Geometry: final body of the model. Coordinates: model frame, mm. Round coordinates to 2 decimals unless told otherwise and drop trailing zeros. Loops run counter-clockwise (first coordinate to the right, second up) from the corner with the lowest first, then second, coordinate; pieces in that order, holes last. Notation, with made-up numbers: M 78,18 L 136,18 A22 ccw 136,25 Z; hole C 69,-30 d3. An arc over 180 degrees is marked long. Answer as a JSON object with one key per item and string values.
from build123d import *

# Parameters (mm, degrees)
SKETCH2_R           = 5
BOSS_EXTRUDE1_DEPTH = 10


with BuildPart() as part:
    # Sketch2 → Boss-Extrude1 (new body)
    with BuildSketch(Plane.XY):
        with BuildLine():
            Line((-737.317762878, -23.619861577), (63.164701196, -23.619861577))
            ThreePointArc((63.164701196, -23.619861577), (70.235769008, -20.690929389), (73.164701196, -13.619861577))
            Line((73.164701196, -13.619861577), (73.164701196, 256.380138423))
            ThreePointArc((73.164701196, 256.380138423), (68.771302914, 266.986740141), (58.164701196, 271.380138423))
            Line((58.164701196, 271.380138423), (-688.827843183, 271.380138423))
            ThreePointArc((-688.827843183, 271.380138423), (-695.25571928, 269.040582854), (-698.675920713, 263.116620199))
            Line((-698.675920713, 263.116620199), (-747.165840408, -11.883379801))
            ThreePointArc((-747.165840408, -11.883379801), (-744.978207309, -20.047737674), (-737.317762878, -23.619861577))
        make_face()
        with Locations(Location((58.164701196, 256.380138423, 0), (0, 0, 180))):
            Circle(SKETCH2_R, mode=Mode.SUBTRACT)
        with Locations((-551.435298804, 26.380138423)):
            Circle(SKETCH2_R, mode=Mode.SUBTRACT)
        with Locations(Location((58.164701196, 26.380138423, 0), (0, 0, 180))):
            Circle(SKETCH2_R, mode=Mode.SUBTRACT)
        with Locations((-551.435298804, 256.380138423)):
            Circle(SKETCH2_R, mode=Mode.SUBTRACT)
        with BuildLine():
            Line((-531.435298804, 46.380138423), (-6.835298804, 46.380138423))
            ThreePointArc((-6.835298804, 46.380138423), (0.235769008, 49.309070611), (3.164701196, 56.380138423))
            Line((3.164701196, 56.380138423), (3.164701196, 136.380138423))
            ThreePointArc((3.164701196, 136.380138423), (0.235769008, 143.451206235), (-6.835298804, 146.380138423))
            Line((-6.835298804, 146.380138423), (-531.435298804, 146.380138423))
            ThreePointArc((-531.435298804, 146.380138423), (-538.506366616, 143.451206235), (-541.435298804, 136.380138423))
            Line((-541.435298804, 136.380138423), (-541.435298804, 56.380138423))
            ThreePointArc((-541.435298804, 56.380138423), (-538.506366616, 49.309070611), (-531.435298804, 46.380138423))
        make_face(mode=Mode.SUBTRACT)
    extrude(amount=BOSS_EXTRUDE1_DEPTH)


solid = part.part
1) Section query B-B (z = 6.5). Return the cut outline in (x, y).
Results:
{"outline": "M -747.17,-11.88 A10 ccw -737.32,-23.62 L 63.16,-23.62 A10 ccw 73.16,-13.62 L 73.16,256.38 A15 ccw 58.16,271.38 L -688.83,271.38 A10 ccw -698.68,263.12 Z; hole C -551.44,26.38 d10; hole C -551.44,256.38 d10; hole M -541.44,56.38 A10 ccw -531.44,46.38 L -6.84,46.38 A10 ccw 3.16,56.38 L 3.16,136.38 A10 ccw -6.84,146.38 L -531.44,146.38 A10 ccw -541.44,136.38 Z; hole C 58.16,26.38 d10; hole C 58.16,256.38 d10"}
2) Section query C-C (y = 113). Return the cut outline in (x, z).
Results:
{"outline": "M -725.15,0 L -541.44,0 L -541.44,10 L -725.15,10 Z; M 3.16,0 L 73.16,0 L 73.16,10 L 3.16,10 Z"}
3) Pin query (flat end, axial travel): P1, Ø9, axis at x = -551.44, y = 256.38, coming from the -Z side; P2, Ø5, axis at y = 113.5, z = 7, coming from the -X side; P3, Ø13, axis at x = -551.44, y = 26.38, coming from the -Z side; P4, Ø3, axis at y = 91, z = 3, coming from the -X side. Return the tip coordinate at first contact, or that it passes through.
Results:
{"P1": "through", "P2": "x = -725.5", "P3": "z = 0", "P4": "x = -729.29"}
4) Section query A-A (x = -383). Return the cut outline in (y, z), and give its area (3 significant figures).
Results:
{"outline": "M -23.62,0 L 46.38,0 L 46.38,10 L -23.62,10 Z; M 146.38,0 L 271.38,0 L 271.38,10 L 146.38,10 Z", "area": "1,950 mm2"}
5) Section query D-D (y = 199.5). Return the cut outline in (x, z), and give its area (3 significant figures).
Results:
{"outline": "M -709.89,0 L 73.16,0 L 73.16,10 L -709.89,10 Z", "area": "7,830 mm2"}
6) Ray query, line 1 (Y direction, x = -394, z = 6); line 2 (X direction, y = 252.5, z = 5.75); line 3 (X direction, y = 253, z = 9.25). Return the intervals inside material, ascending.
Results:
{"line 1": "-23.62 to 46.38, 146.38 to 271.38", "line 2": "-700.55 to -554.59, -548.28 to 55.01, 61.32 to 73.16", "line 3": "-700.46 to -555.12, -547.75 to 54.48, 61.85 to 73.16"}
